```python
from build123d import *

# Parameters (mm, degrees)
SKETCH_1_R      = 1.5
SKETCH_1_W      = 8.2
SKETCH_1_H      = 2.2
SKETCH_1_W_2    = 2.2
SKETCH_1_H_2    = 8.2
SKETCH_1_R_2    = 3
EXTRUDE_1_DEPTH = 2


with BuildPart() as part:
    # 草图1 → 凸台-拉伸1 (new body)
    with BuildSketch(Plane.XY):
        Polygon((-68.061769393, -13.095981945), (-52.184883937, -13.095981945), (-18.934883937, -13.095981945), (18.565116063, -13.095981945), (67.695116063, -13.095981945), (171.815116063, 33.779018055), (171.815116063, 73.779018055), (114.815116063, 73.779018055), (114.815116063, 71.279018055), (116.315116063, 71.279018055), (116.315116063, 68.679018055), (114.815116063, 68.679018055), (114.815116063, 65.679018055), (111.815116063, 65.679018055), (111.815116063, 68.679018055), (110.315116063, 68.679018055), (110.315116063, 71.279018055), (111.815116063, 71.279018055), (111.815116063, 73.779018055), (1.315116063, 73.779018055), (1.315116063, 71.279018055), (2.815116063, 71.279018055), (2.815116063, 68.679018055), (1.315116063, 68.679018055), (1.315116063, 65.679018055), (-1.684883937, 65.679018055), (-1.684883937, 68.679018055), (-3.184883937, 68.679018055), (-3.184883937, 71.279018055), (-1.684883937, 71.279018055), (-1.684883937, 73.779018055), (-68.061769393, 73.779018055), align=None)
        with Locations((-33.184883937, -9.095981945)):
            Circle(SKETCH_1_R, mode=Mode.SUBTRACT)
        with Locations((-17.934883937, -9.095981946)):
            Rectangle(SKETCH_1_W, SKETCH_1_H, mode=Mode.SUBTRACT)
        with Locations((17.565116063, -9.095981946)):
            Rectangle(SKETCH_1_W, SKETCH_1_H, mode=Mode.SUBTRACT)
        with Locations((32.815116063, -9.095981945)):
            Circle(SKETCH_1_R, mode=Mode.SUBTRACT)
        with Locations((-64.184883937, 22.341518055)):
            Rectangle(SKETCH_1_W_2, SKETCH_1_H_2, mode=Mode.SUBTRACT)
        with Locations((63.815116063, 22.341518055)):
            Rectangle(SKETCH_1_W_2, SKETCH_1_H_2, mode=Mode.SUBTRACT)
        with BuildLine():
            ThreePointArc((50.815116063, 61.279018055), (52.936436406, 60.400338398), (53.815116063, 58.279018055))
            Line((53.815116063, 58.279018055), (53.815116063, 2.904018055))
            ThreePointArc((53.815116063, 2.904018055), (52.936436406, 0.782697711), (50.815116063, -0.095981945))
            Line((50.815116063, -0.095981945), (-51.184883937, -0.095981945))
            ThreePointArc((-51.184883937, -0.095981945), (-53.306204281, 0.782697711), (-54.184883937, 2.904018055))
            Line((-54.184883937, 2.904018055), (-54.184883937, 58.279018055))
            ThreePointArc((-54.184883937, 58.279018055), (-53.306204281, 60.400338398), (-51.184883937, 61.279018055))
            Line((-51.184883937, 61.279018055), (50.815116063, 61.279018055))
        make_face(mode=Mode.SUBTRACT)
        with Locations((-64.184883937, 53.779018055)):
            Circle(SKETCH_1_R, mode=Mode.SUBTRACT)
        Polygon((139.815116063, 48.679018055), (124.815116063, 48.679018055), (101.815116063, 48.679018055), (101.815116063, 58.879018055), (124.815116063, 58.879018055), (139.815116063, 58.879018055), align=None, mode=Mode.SUBTRACT)
        with Locations((149.815116063, 53.779018055)):
            Circle(SKETCH_1_R_2, mode=Mode.SUBTRACT)
    extrude(amount=EXTRUDE_1_DEPTH)


solid = part.part
```
CAD build for the part. Positions are in the model's coordinates, mm. Round coordinates to 2 decimals unless told otherwise and drop trailing zeros. Write each loop counter-clockwise with the first axis right and the second up, starting at its lowest first coordinate (ties: lowest second). Pieces come first, ordered by that corner, then holes. Notation, with made-up numbers: (77, -5.5) - (88, -5.5) arc R21 ccw to (88, 32.5) - close; hole circle Ø7 at (39, 84). An arc over 180 degrees is marked (long way). Write item = value, one per line. Start each with the question number.
Q1. Drop a flat-ended pin along its axis: pin 1 (3 mm diameter, centred on x = 61.5, y = 41.5, fed in from -Z). Give the stop position or say it passes through.
Q2. Band-saw the part on C-C (y = 24). Give the cut face in (x, z).
Q3. Band-saw the part on A-A (y = 44). Give the cut face in (x, z).
Q4. Band-saw the part on D-D (z = 1.35). Count the separate pieces of the cut face and the enclosed holes in it, then the cut area to 3 significant figures.
Q5. Band-saw the part on B-B (x = -24.5). Give the cut face in (y, z), then the cut area to 3 significant figures.
Q6. Mould opens along Y. For faces 1 (the cylindrical face through (152.677, 54.68, 0.986)), 2 (the flat face through (119, 10, 1)), 3 (the flat face through (77, 31, 0)) say: pulls with the +Y half, pulls with the -Y half, needs draft (parallel to the pull), parting line crosses it, or undercut.
Q7. Probe L1, parallel to X at y = 57.5, z = 0.15; L2, parallel to X at y = 40.5, z = 0.35; L3, parallel to Y at x = 50, z = 0.9. List the from-to ranges inside material, lowest first. Write a range as from..to.
Answers below:
q1.pin_1 = 0
q2.outline = (-68.06, 0) - (-65.28, 0) - (-65.28, 2) - (-68.06, 2) - close; (-63.08, 0) - (-54.18, 0) - (-54.18, 2) - (-63.08, 2) - close; (53.82, 0) - (62.72, 0) - (62.72, 2) - (53.82, 2) - close; (64.92, 0) - (150.09, 0) - (150.09, 2) - (64.92, 2) - close
q3.outline = (-68.06, 0) - (-54.18, 0) - (-54.18, 2) - (-68.06, 2) - close; (53.82, 0) - (171.82, 0) - (171.82, 2) - (53.82, 2) - close
q4.separate_pieces = 1
q4.enclosed_holes = 10
q4.area = 11,200 mm2
q5.outline = (-13.1, 0) - (-0.1, 0) - (-0.1, 2) - (-13.1, 2) - close; (61.28, 0) - (73.78, 0) - (73.78, 2) - (61.28, 2) - close
q5.area = 51.0 mm2
q6.face_1 = undercut
q6.face_2 = pulls with the -Y half
q6.face_3 = needs draft
q7.L1 = -68.06..-54.18, 53.82..101.82, 139.82..171.82
q7.L2 = -68.06..-54.18, 53.82..171.82
q7.L3 = -13.1..-0.1, 61.28..73.78
